```python
from build123d import *

# Parameters (mm, degrees)
SKETCH1_W           = 74
SKETCH1_H           = 13
SKETCH1_R           = 2
BOSS_EXTRUDE1_DEPTH = 2
SKETCH2_W           = 2
SKETCH2_H           = 9.5775
SKETCH2_W_2         = 1
SKETCH2_H_2         = 1
BOSS_EXTRUDE2_DEPTH = 8
SKETCH3_W           = 12
SKETCH3_H           = 19
BOSS_EXTRUDE3_DEPTH = 4
FILLET1_R           = 0.5


with BuildPart() as part:
    # Sketch1 → Boss-Extrude1 (new body)
    with BuildSketch(Plane(origin=(0, 0, 0), x_dir=(1, 0, 0), z_dir=(0, 1, 0))):
        Rectangle(SKETCH1_W, SKETCH1_H)
        with Locations(Location((-33.5, -3, 0), (0, 0, 270))):
            Circle(SKETCH1_R, mode=Mode.SUBTRACT)
        with Locations(Location((33.5, -3, 0), (0, 0, 90))):
            Circle(SKETCH1_R, mode=Mode.SUBTRACT)
    extrude(amount=BOSS_EXTRUDE1_DEPTH)

    # Sketch2 → Boss-Extrude2 (add)
    # profile 1 of 2: a face of its own
    with BuildSketch(Plane(origin=(0, 2, 0), x_dir=(1, 0, 0), z_dir=(0, 1, 0))):
        with Locations((11, 1.51125)):
            Rectangle(SKETCH2_W, SKETCH2_H)
        with Locations((11, 2.774166667)):
            Rectangle(SKETCH2_W_2, SKETCH2_H_2, mode=Mode.SUBTRACT)
        with Locations((11, 5.3)):
            Rectangle(SKETCH2_W_2, SKETCH2_H_2, mode=Mode.SUBTRACT)
        with Locations((11, 0.248333333)):
            Rectangle(SKETCH2_W_2, SKETCH2_H_2, mode=Mode.SUBTRACT)
        with Locations((11, -2.2775)):
            Rectangle(SKETCH2_W_2, SKETCH2_H_2, mode=Mode.SUBTRACT)
    # profile 2 of 2: a face of its own
    with BuildSketch(Plane(origin=(0, 2, 0), x_dir=(1, 0, 0), z_dir=(0, 1, 0))):
        with Locations((-15, 1.51125)):
            Rectangle(SKETCH2_W, SKETCH2_H)
        with Locations((-15, -2.2775)):
            Rectangle(SKETCH2_W_2, SKETCH2_H_2, mode=Mode.SUBTRACT)
        with Locations((-15, 0.248333333)):
            Rectangle(SKETCH2_W_2, SKETCH2_H_2, mode=Mode.SUBTRACT)
        with Locations((-15, 2.774166667)):
            Rectangle(SKETCH2_W_2, SKETCH2_H_2, mode=Mode.SUBTRACT)
        with Locations((-15, 5.3)):
            Rectangle(SKETCH2_W_2, SKETCH2_H_2, mode=Mode.SUBTRACT)
    extrude(amount=BOSS_EXTRUDE2_DEPTH)

    # Sketch3 → Boss-Extrude3 (add)
    with BuildSketch(Plane(origin=(0, 0.75, 0), x_dir=(1, 0, 0), z_dir=(0, 1, 0))):
        with Locations((-1, 12)):
            Rectangle(SKETCH3_W, SKETCH3_H)
    extrude(amount=BOSS_EXTRUDE3_DEPTH)

    # Fillet1
    fillet1_edges = [part.edges().sort_by_distance(p)[0] for p in [
        (5, 0.75, -14),
        (-7, 0.75, -14),
        (5, 4.75, -12),
        (-7, 4.75, -12),
    ]]
    fillet(fillet1_edges, radius=FILLET1_R)


solid = part.part
```
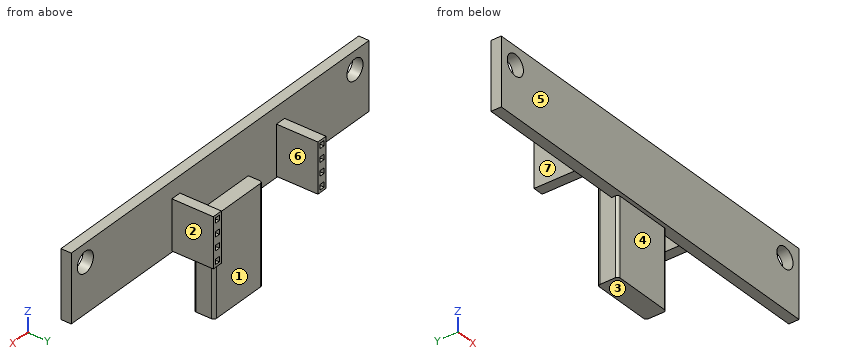
Could you check a few things on this model? Use its own coordinates, in mm. Face numbers are marked on the shaded views. A direction names the side the tool comes from. Coordinates: 2 decimals unless noted, no trailing zeros. Write each loop counter-clockwise with the first axis right and the second up, starting at its lowest first coordinate (ties: lowest second). Pieces come first, ordered by that corner, then holes. Notation, with made-up numbers: (-22, -3.5) -> (34, -3.5) arc R30 ccw to (34, 23.5) -> close; hole circle Ø9 at (88, 61.5). An arc over 180 degrees is marked (long way). Write item = value, one per line. Start each with the question number.
(1) Will these pins go through, and if not, where does the flat tip stop? pin 1 (0.8 mm diameter, centred on y = 5, z = -0.5, fed in from +X); pin 2 (1 mm diameter, centred on x = 10.5, y = 7.5, fed in from -Z); pin 3 (2 mm diameter, centred on x = 10.5, y = 7, fed in from +Z); pin 4 (4 mm diameter, centred on y = 8, z = -12.5, fed in from +X).
(2) I want a section at B-B (z = -9.75). Please give me the cut outline in (x, y).
(3) I want a section at D-D (x = 7.5). Please give me the cut outline in (y, z), plus the area to 3 significant figures.
(4) Which directions (+Z, -Z, +X, -X, +Y, -Y) give clear straight access to the entire face, cutting with the end or side of a thin tool? Please do the marked faces 1, 2, 3 and 4.
(5) I want a section at A-A (x = -33.5). Please give me the cut outline in (y, z), plus the area to 3 significant figures.
(6) I need wall thicknesses on line 1 (X direction, y = 1.6, z = 3); line 2 (X direction, y = 2.5, z = -3); line 3 (X direction, y = 5.5, z = 2). Which ranges of each line are inside material? Lowest first, please. Write a range as [from, to].
(7) I want a section at C-C (y = 3). Give the number of separate pieces and of enclosed holes in the cut face, plus the area to 3 significant figures.
(8) We'd pull the mould along X, two halves only. Please class the marked faces 5, 6 and 7: released by +X, released by -X, zero draft, split by the parting line, or undercut.
Result set:
q1.pin_1 = 12
q1.pin_2 = -6.3
q1.pin_3 = 3.28
q1.pin_4 = through
q2.outline = (-7, 1.25) arc R0.5 ccw to (-6.5, 0.75) -> (4.5, 0.75) arc R0.5 ccw to (5, 1.25) -> (5, 4.25) arc R0.5 ccw to (4.5, 4.75) -> (-6.5, 4.75) arc R0.5 ccw to (-7, 4.25) -> close
q3.outline = (0, -6.5) -> (2, -6.5) -> (2, 6.5) -> (0, 6.5) -> close
q3.area = 26.0 mm2
q4.face_1 = +Z, -Z, +Y
q4.face_2 = +Z, -Z, +X, +Y
q4.face_3 = -Z, +X, -X, +Y, -Y
q4.face_4 = -Z, +X, -X, -Y
q5.outline = (0, -6.5) -> (2, -6.5) -> (2, 1) -> (0, 1) -> close; (0, 5) -> (2, 5) -> (2, 6.5) -> (0, 6.5) -> close
q5.area = 18.0 mm2
q6.line_1 = [-37, -35.5], [-31.5, 31.5], [35.5, 37]
q6.line_2 = [-16, -15.5], [-14.5, -14], [-7, 5], [10, 10.5], [11.5, 12]
q6.line_3 = [-16, -15.5], [-14.5, -14], [10, 10.5], [11.5, 12]
q7.separate_pieces = 3
q7.enclosed_holes = 8
q7.area = 258 mm2
q8.face_5 = zero draft
q8.face_6 = undercut
q8.face_7 = released by -X
